Could you check a few things on this model? Use its own coordinates, in mm. A direction names the side the tool comes from. Give positions to 0.01 mm unless a question says otherwise; leave off trailing zeros. Write each loop counter-clockwise with the first axis right and the second up, starting at its lowest first coordinate (ties: lowest second). Pieces come first, ordered by that corner, then holes. Notation, with made-up numbers: (77, 6.25) - (130, 6.25) arc R30 ccw to (130, 39.25) - close; hole circle Ø8 at (-7.5, 16.5). An arc over 180 degrees is marked (long way). Answer as a JSON object with one key per item and string values. Group by question number.
```python
from build123d import *

# Parameters (mm, degrees)
SKETCH_1_W      = 650
SKETCH_1_H      = 252
SKETCH_1_W_2    = 600
SKETCH_1_H_2    = 202
EXTRUDE_1_DEPTH = 7.5
SKETCH_2_W      = 600
SKETCH_2_H      = 202
EXTRUDE_2_DEPTH = 2.5


with BuildPart() as part:
    # 草图1 → 凸台-拉伸1 (new body, symmetric)
    with BuildSketch(Plane(origin=(0, 0, 0), x_dir=(1, 0, 0), z_dir=(0, 1, 0))):
        Rectangle(SKETCH_1_W, SKETCH_1_H)
        Rectangle(SKETCH_1_W_2, SKETCH_1_H_2, mode=Mode.SUBTRACT)
    extrude(amount=EXTRUDE_1_DEPTH, both=True)

    # 草图2 → 凸台-拉伸2 (add, symmetric)
    with BuildSketch(Plane(origin=(0, 0, 0), x_dir=(1, 0, 0), z_dir=(0, 1, 0))):
        Rectangle(SKETCH_2_W, SKETCH_2_H)
    extrude(amount=EXTRUDE_2_DEPTH, both=True)


solid = part.part
```
(1) If we mould it in two halves opening along X, with no side actions, what happens to faces 1 (the flat face through (-4, -2.5, -1)), 2 (the flat face through (-5, 0, 126)), 3 (the flat face through (-325, 0, 2))? For each: +X half, -X half, draft (parallel to the pull), parting line (faces both ways), or undercut.
(2) I need wall thicknesses on L1, parallel to X at y = -6.75, z = 87.5; L2, parallel to Z at x = -37.5, y = -7; L3, parallel to Y at x = -180, z = -64. Which ranges of each line are inside material? Lowest first, please.
(3) I want a section at C-C, the plane z = -35.5. Please give me the cut outline in (x, y), and give its area (3 significant figures).
(4) I want a section at B-B, the plane x = 271. Please give me the cut outline in (y, z), and give its area (3 significant figures).
(5) Will these pins go through, and if not, where does the flat tip stop? P1, Ø4, axis at x = 52.5, z = 55.5, coming from the -Y side; P2, Ø2, axis at x = 214, z = 48.5, coming from the +Y side.
(6) For faces 4 (the flat face through (-4, 2.5, -1)), 5 (the flat face through (-26, -7.5, 102)), which set-ups out of +Z, -Z, +X, -X, +Y, -Y let a thin tool reach every point of the face, with its end or its side?
(7) I want a section at A-A, the plane y = 5. Please give me the cut outline in (x, z), and give its area (3 significant figures).
Entries:
{
 "1": {"face 1": "undercut", "face 2": "draft", "face 3": "-X half"},
 "2": {"L1": "-325 to -300, 300 to 325", "L2": "-126 to -101, 101 to 126", "L3": "-2.5 to 2.5"},
 "3": {"outline": "(-325, -7.5) - (-300, -7.5) - (-300, -2.5) - (300, -2.5) - (300, -7.5) - (325, -7.5) - (325, 7.5) - (300, 7.5) - (300, 2.5) - (-300, 2.5) - (-300, 7.5) - (-325, 7.5) - close", "area": "3,750 mm^2"},
 "4": {"outline": "(-7.5, -126) - (7.5, -126) - (7.5, -101) - (2.5, -101) - (2.5, 101) - (7.5, 101) - (7.5, 126) - (-7.5, 126) - (-7.5, 101) - (-2.5, 101) - (-2.5, -101) - (-7.5, -101) - close", "area": "1,760 mm^2"},
 "5": {"P1": "y = -2.5", "P2": "y = 2.5"},
 "6": {"face 4": "+Y", "face 5": "+Z, -Z, +X, -X, -Y"},
 "7": {"outline": "(-325, -126) - (325, -126) - (325, 126) - (-325, 126) - close; hole (-300, -101) - (300, -101) - (300, 101) - (-300, 101) - close", "area": "42,600 mm^2"}
}
